Input: dimensioned drawing with shaded views. Units: mm. Origin: part minimum x, y, z. Give positions to 0.01 mm unless a question says otherwise; leave off trailing zeros. Write each loop counter-clockwise with the first axis right and the second up, starting at its lowest first coordinate (ties: lowest second). Pieces come first, ordered by that corner, then holes. Notation, with made-up numbers: M 56.5,-39.5 L 86.5,-39.5 A21 ccw 86.5,-35.5 Z; hole C 86,-5.75 d4. An arc over 180 degrees is marked long. Use CSV: the item, a comma, the result in double quotes. Start each with the question number.
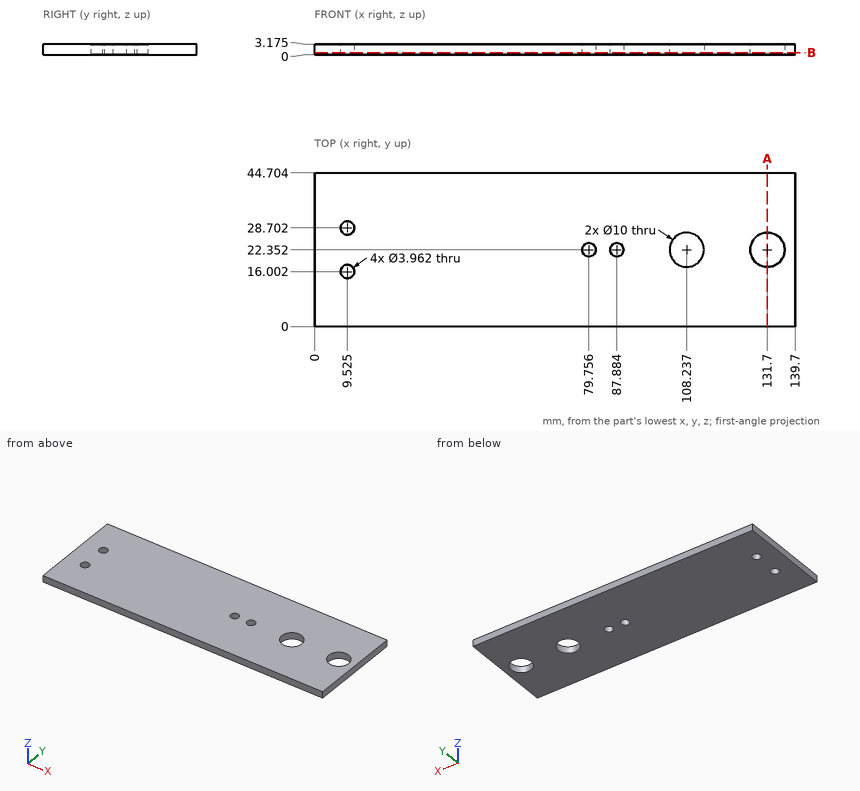
Item 1: Section A-A (x = 131.7). Return the cut outline in (y, z) (1 decimal).
Item 2: Contact query for a flat-ended pin moving along its axis: pin 1 Ø1 at (x, z) = (93, 2) entering from -Y. Output: stop coordinate, or through.
Item 3: Section B-B (z = 0.65). Return the cut outline in (x, y) (1 decimal).
Item 4: Material intervals for probe 1 along X at (y, z) = (29, 2.4); probe 2 along Y at (x, z) = (129, 1.9) (1 decimal); probe 3 along Y at (x, z) = (128, 3) (1 decimal), sorted ascending.
Output values:
1,outline,"M 0,0 L 17.4,0 L 17.4,3.2 L 0,3.2 Z; M 27.4,0 L 44.7,0 L 44.7,3.2 L 27.4,3.2 Z"
2,pin 1,"stops at y = 0"
3,outline,"M 0,0 L 139.7,0 L 139.7,44.7 L 0,44.7 Z; hole C 9.5,16 d4; hole C 9.5,28.7 d4; hole C 79.8,22.4 d4; hole C 87.9,22.4 d4; hole C 108.2,22.4 d10; hole C 131.7,22.4 d10"
4,probe 1,"x = 0 to 7.57, 11.48 to 139.7"
4,probe 2,"y = 0 to 18.1, 26.6 to 44.7"
4,probe 3,"y = 0 to 19, 25.7 to 44.7"
